The model under review builds one solid part; all positions refer to its coordinate system, in mm. Round coordinates to 2 decimals unless told otherwise and drop trailing zeros. Loops run counter-clockwise (first coordinate to the right, second up) from the corner with the lowest first, then second, coordinate; pieces in that order, holes last. Notation, with made-up numbers: M 42.25,88.5 L 57.25,88.5 A20 ccw 57.25,95.5 Z; hole C 37.5,75 d1. An arc over 180 degrees is marked long. Answer as a JSON object with one key per item and string values. Group by question number.
Item 1: Consider section B-B (z = 9). Give the boundary of the cut face in (x, y).
Item 2: Insertion check: P1, Ø5, axis at x = -11, y = 3, coming from the +Z side; P2, Ø3.5, axis at x = 8, z = -8, coming from the +Y side; P3, Ø3, axis at y = 1.5, z = 12.5, coming from the -X side; P4, Ø5, axis at y = 9.5, z = -5, coming from the +X side. Each pin has a flat end and moves straight along its axis. Give the tip position at first contact, or say it passes through.
Item 3: Consider section A-A (x = 9). Give the boundary of the cut face in (y, z).
Item 4: Consider section C-C (y = 5.75). Give the boundary of the cut face in (x, z), and give its area (3 significant figures).
Item 5: The part is to be moulded in two halves that separate along X. For faces 1 (the face through (-15.213, 6.212, -4.791)), 2 (the face through (0, 0, 0)), 3 (the face through (8.273, 6.212, 5.918)), say which applies: +X half, -X half, draft (parallel to the pull), parting line (faces both ways), or undercut.
Item 6: To check wall thickness, follow line 1 (X direction, y = 7.75, z = 7); line 2 (Z direction, x = 6.5, y = 1); line 3 (X direction, y = 2, z = -9). State the ranges of each line that lie inside material, in increasing order.
Item 7: Consider section D-D (x = 13). Give the boundary of the cut face in (y, z).
Autodesk Inventor part; units mm, degrees
ref_plane "YZ Plane" through (0, 0, 0) normal (1, 0, 0) x (0, 1, 0)
ref_plane "XZ Plane" through (0, 0, 0) normal (0, 1, 0) x (-1, 0, 0)
ref_plane "XY Plane" through (0, 0, 0) normal (0, 0, 1) x (1, 0, 0)
sketch "Sketch1" plane through (0, 0, 0) normal (0, 1, 0) x (-1, 0, 0)
  circle A0 centre (0, 0) radius 15.95
  circle A1 centre (8, 8) radius 2.1
  circle A2 centre (-8, 8) radius 2.1
  circle A3 centre (-8, -8) radius 2.1
  circle A4 centre (8, -8) radius 2.1
  dimension "d0" = 31.9
  dimension "d1" = 4.2
  dimension "d2" = 8
  dimension "d3" = 8
  dimension "d6" = 360
extrude "Extrusion1" add sketch "Sketch1" along normal blind 12.6
properties part number "EndEffector_Stage1BearingSpacer" material "Aluminum 6061"
Geometry results:
{
 "1": {"outline": "M -13.17,0 L -9.85,0 L -9.85,12.6 L -13.17,12.6 Z; M -6.15,0 L 6.15,0 L 6.15,12.6 L -6.15,12.6 Z; M 9.85,0 L 13.17,0 L 13.17,12.6 L 9.85,12.6 Z"},
 "2": {"P1": "stops at z = 13.5", "P2": "passes through", "P3": "stops at x = -11.55", "P4": "stops at x = 15.75"},
 "3": {"outline": "M 0,-13.17 L 12.6,-13.17 L 12.6,-9.85 L 0,-9.85 Z; M 0,-6.15 L 12.6,-6.15 L 12.6,6.15 L 0,6.15 Z; M 0,9.85 L 12.6,9.85 L 12.6,13.17 L 0,13.17 Z"},
 "4": {"outline": "C 0,0 d31.9; hole C -8,-8 d4.2; hole C -8,8 d4.2; hole C 8,-8 d4.2; hole C 8,8 d4.2", "area": "744 mm^2"},
 "5": {"face 1": "parting line", "face 2": "draft", "face 3": "undercut"},
 "6": {"line 1": "x = -14.33 to -9.85, -6.15 to 6.15, 9.85 to 14.33", "line 2": "z = -14.57 to -9.47, -6.53 to 6.53, 9.47 to 14.57", "line 3": "x = -13.17 to -9.85, -6.15 to 6.15, 9.85 to 13.17"},
 "7": {"outline": "M 0,-9.24 L 12.6,-9.24 L 12.6,9.24 L 0,9.24 Z"}
}
